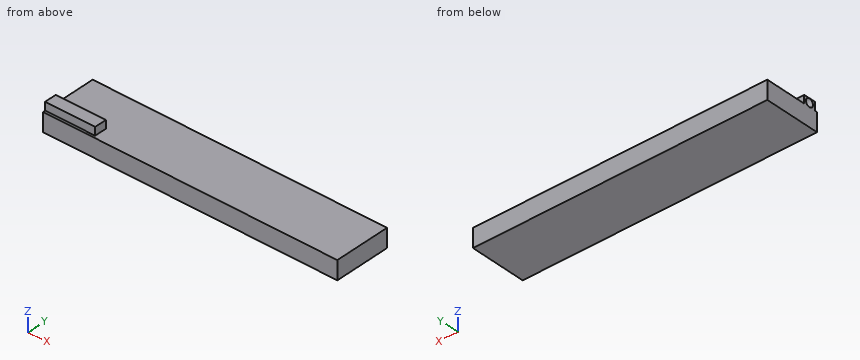
from build123d import *

# Parameters (mm, degrees)
SKETCH1_W           = 36.5
SKETCH1_H           = 7
BOSS_EXTRUDE1_DEPTH = 2.3
SKETCH2_W           = 6.2
SKETCH2_H           = 1.5
BOSS_EXTRUDE2_DEPTH = 1
SKETCH3_R           = 0.5
CUT_EXTRUDE1_DEPTH  = 1


with BuildPart() as part:
    # Sketch1 → Boss-Extrude1 (new body)
    with BuildSketch(Plane.XY):
        with Locations((18.25, -3.5)):
            Rectangle(SKETCH1_W, SKETCH1_H)
    extrude(amount=BOSS_EXTRUDE1_DEPTH)

    # Sketch2 → Boss-Extrude2 (add)
    with BuildSketch(Plane.XY.offset(2.3)):
        with Locations((3.1, -5.95)):
            Rectangle(SKETCH2_W, SKETCH2_H)
    extrude(amount=BOSS_EXTRUDE2_DEPTH)

    # Sketch3 → Cut-Extrude1 (cut)
    with BuildSketch(Plane.ZY):
        with Locations(Location((2.779912682, -5.934327953, 0), (0, 0, 270))):
            Circle(SKETCH3_R)
    extrude(amount=-CUT_EXTRUDE1_DEPTH, mode=Mode.SUBTRACT)


solid = part.part
Model file for the job. Use its own axes, mm. Give positions to 0.01 mm unless a question says otherwise; leave off trailing zeros. Loops run counter-clockwise (first coordinate to the right, second up) from the corner with the lowest first, then second, coordinate; pieces in that order, holes last. Notation, with made-up numbers: (72.25, 19) - (107.25, 19) arc R17 cw to (107.25, 30) - close; hole circle Ø6 at (75.5, 57.25). An arc over 180 degrees is marked (long way). Use one line per item in the form item = value.
(1) Drop flat-ended pins along their axis: P1, Ø1.5, axis at x = 8.5, y = -4.5, coming from the +Z side; P2, Ø1.1, axis at y = -5.5, z = 3, coming from the +X side; P3, Ø0.8, axis at x = 4, z = 3, coming from the -Y side. Give the stop position or say it passes through.
Determined:
P1 = 2.3
P2 = 6.2
P3 = -6.7
(2) Drill centre lines: L1, parallel to Z at x = 14, y = -6.5; L2, parallel to X at y = -6, z = 2.95; L3, parallel to Y at x = 4, z = 2.7. Where is each one in solid material? Low to high.
Determined:
L1 = 0 to 2.3
L2 = 1 to 6.2
L3 = -6.7 to -5.2
(3) Cut at B-B (y = -3.75). Give the cut face in (x, z), then the cut area to 4 significant figures.
Determined:
outline = (0, 0) - (36.5, 0) - (36.5, 2.3) - (0, 2.3) - close
area = 83.95 mm^2
(4) Cut at A-A (x = 12). Give the cut face in (y, z).
Determined:
outline = (-7, 0) - (0, 0) - (0, 2.3) - (-7, 2.3) - close
